from build123d import *

# Parameters (mm, degrees)
SKETCH1_R           = 32
SKETCH1_R_2         = 6
BOSS_EXTRUDE1_DEPTH = 0.3


with BuildPart() as part:
    # Sketch1 → Boss-Extrude1 (new body)
    with BuildSketch(Plane(origin=(0, 0, 0), x_dir=(1, 0, 0), z_dir=(0, 1, 0))):
        Circle(SKETCH1_R)
        Circle(SKETCH1_R_2, mode=Mode.SUBTRACT)
        with BuildLine():
            ThreePointArc((0, 25.5), (-25.112597702, 4.428028531), (-8.721513655, -23.96216183))
            ThreePointArc((-8.721513655, -23.96216183), (-8.080657273, -23.663325591), (-8.379493511, -23.022469209))
            ThreePointArc((-8.379493511, -23.022469209), (-24.127789949, 4.254380353), (0, 24.5))
            ThreePointArc((0, 24.5), (0.5, 25), (0, 25.5))
        make_face(mode=Mode.SUBTRACT)
        with BuildLine():
            ThreePointArc((18.5, 0), (3.212491287, 18.218943431), (-17.384313485, 6.327372652))
            ThreePointArc((-17.384313485, 6.327372652), (-17.085477246, 5.686516269), (-16.444620864, 5.985352508))
            ThreePointArc((-16.444620864, 5.985352508), (3.038843109, 17.234135678), (17.5, 0))
            ThreePointArc((17.5, 0), (18, -0.5), (18.5, 0))
        make_face(mode=Mode.SUBTRACT)
        with BuildLine():
            ThreePointArc((0, -25.5), (25.112597702, -4.428028531), (8.721513655, 23.96216183))
            ThreePointArc((8.721513655, 23.96216183), (8.080657273, 23.663325591), (8.379493511, 23.022469209))
            ThreePointArc((8.379493511, 23.022469209), (24.127789949, -4.254380353), (0, -24.5))
            ThreePointArc((0, -24.5), (-0.5, -25), (0, -25.5))
        make_face(mode=Mode.SUBTRACT)
        with BuildLine():
            ThreePointArc((0, 11.5), (-11.32528916, 1.996954043), (-3.933231648, -10.806465139))
            ThreePointArc((-3.933231648, -10.806465139), (-3.292375266, -10.5076289), (-3.591211505, -9.866772518))
            ThreePointArc((-3.591211505, -9.866772518), (-10.340481407, 1.823305866), (0, 10.5))
            ThreePointArc((0, 10.5), (0.5, 11), (0, 11.5))
        make_face(mode=Mode.SUBTRACT)
        with BuildLine():
            ThreePointArc((0, -11.5), (11.32528916, -1.996954043), (3.933231648, 10.806465139))
            ThreePointArc((3.933231648, 10.806465139), (3.292375266, 10.5076289), (3.591211505, 9.866772518))
            ThreePointArc((3.591211505, 9.866772518), (10.340481407, -1.823305866), (0, -10.5))
            ThreePointArc((0, -10.5), (-0.5, -11), (0, -11.5))
        make_face(mode=Mode.SUBTRACT)
        with BuildLine():
            ThreePointArc((-18.5, 0), (-3.212491287, -18.218943431), (17.384313485, -6.327372652))
            ThreePointArc((17.384313485, -6.327372652), (17.085477246, -5.686516269), (16.444620864, -5.985352508))
            ThreePointArc((16.444620864, -5.985352508), (-3.038843109, -17.234135678), (-17.5, 0))
            ThreePointArc((-17.5, 0), (-18, 0.5), (-18.5, 0))
        make_face(mode=Mode.SUBTRACT)
    extrude(amount=BOSS_EXTRUDE1_DEPTH)


solid = part.part
Input: part model. Units: mm. Frame: model coordinates. A direction names the side the tool comes from. Give positions to 0.01 mm unless a question says otherwise; leave off trailing zeros. Write each loop counter-clockwise with the first axis right and the second up, starting at its lowest first coordinate (ties: lowest second). Pieces come first, ordered by that corner, then holes.
Q1. Pull-direction query (Z, two-part tool) for faces 3 (the face through (7, 0.3, 0)), 4 (the face through (-4.76, 0.15, 3.65)), 5 (the face through (-6.94, 0.15, 31.24)); classes: pulls with the +Z half, pulls with the -Z half, needs draft (parallel to the pull), parting line crosses it, or undercut.
Q2. Section D-D, the plane x = 22. Output: boundary loops of the cut face in (y, z).
Q3. Section B-B, the plane x = 14. Output: boundary loops of the cut face in (y, z).
Q4. Section C-C, the plane y = 0.05. Output: boundary loops of the cut face in (x, z).
Q5. Material intervals for probe 1 along X at (y, z) = (0.2, -16); probe 2 along X at (y, z) = (0.2, -13); probe 3 along Z at (x, y) = (-7, 0.1), sorted ascending.
Q6. Section A-A, the plane z = -8.5. Output: boundary loops of the cut face in (x, y), plus the area to 3 significant figures.
Q7. Set-up query: faces 1 (the face through (-25.02, 0.15, -4.92)), 2 (the face through (7, 0, 0)). Return all of +Z, -Z, +X, -X, +Y, -Y with unobstructed straight access to the full face (end or side cutting, diameter ignored); none if empty.
Filled in:
1. face 3: needs draft
1. face 4: undercut
1. face 5: parting line crosses it
2. outline: (0, -23.24) - (0.3, -23.24) - (0.3, -12.89) - (0, -12.89) - close; (0, -10.78) - (0.3, -10.78) - (0.3, 10.78) - (0, 10.78) - close; (0, 12.89) - (0.3, 12.89) - (0.3, 23.24) - (0, 23.24) - close
3. outline: (0, -28.77) - (0.3, -28.77) - (0.3, -21.31) - (0, -21.31) - close; (0, -20.11) - (0.3, -20.11) - (0.3, -12.09) - (0, -12.09) - close; (0, -10.5) - (0.3, -10.5) - (0.3, 10.5) - (0, 10.5) - close; (0, 12.09) - (0.3, 12.09) - (0.3, 20.11) - (0, 20.11) - close; (0, 21.31) - (0.3, 21.31) - (0.3, 28.77) - (0, 28.77) - close
4. outline: circle Ø64 at (0, 0); hole (-18.5, 0) arc R0.5 ccw to (-17.5, 0) arc R17.5 cw to (16.44, 5.99) arc R0.5 ccw to (17.38, 6.33) arc R18.5 ccw to start; hole (-17.38, -6.33) arc R18.5 ccw to (18.5, 0) arc R0.5 ccw to (17.5, 0) arc R17.5 cw to (-16.44, -5.99) arc R0.5 ccw to start; hole (-8.72, 23.96) arc R25.5 ccw to (0, -25.5) arc R0.5 ccw to (0, -24.5) arc R24.5 cw to (-8.38, 23.02) arc R0.5 ccw to start; hole circle Ø12 at (0, 0); hole (-3.93, 10.81) arc R11.5 ccw to (0, -11.5) arc R0.5 ccw to (0, -10.5) arc R10.5 cw to (-3.59, 9.87) arc R0.5 ccw to start; hole (0, 10.5) arc R10.5 cw to (3.59, -9.87) arc R0.5 ccw to (3.93, -10.81) arc R11.5 ccw to (0, 11.5) arc R0.5 ccw to start; hole (0, 24.5) arc R24.5 cw to (8.38, -23.02) arc R0.5 ccw to (8.72, -23.96) arc R25.5 ccw to (0, 25.5) arc R0.5 ccw to start
5. probe 1: x = -27.71 to -19.86, -18.55 to -9.29, -7.09 to 7.09, 9.29 to 18.55, 19.86 to 27.71
5. probe 2: x = -29.24 to -21.94, -20.77 to -13.16, -11.72 to 11.72, 13.16 to 20.77, 21.94 to 29.24
5. probe 3: z = -31.22 to -24.52, -23.48 to -17.12, -16.04 to -9.12, -7.83 to 7.83, 9.12 to 16.04, 17.12 to 31.22
6. outline: (-30.85, 0) - (-24.04, 0) - (-24.04, 0.3) - (-30.85, 0.3) - close; (-22.98, 0) - (-16.43, 0) - (-16.43, 0.3) - (-22.98, 0.3) - close; (-15.3, 0) - (-7.75, 0) - (-7.75, 0.3) - (-15.3, 0.3) - close; (-6.16, 0) - (6.16, 0) - (6.16, 0.3) - (-6.16, 0.3) - close; (7.75, 0) - (15.3, 0) - (15.3, 0.3) - (7.75, 0.3) - close; (16.43, 0) - (22.98, 0) - (22.98, 0.3) - (16.43, 0.3) - close; (24.04, 0) - (30.85, 0) - (30.85, 0.3) - (24.04, 0.3) - close
6. area: 16.2 mm2
7. face 1: +Y, -Y
7. face 2: +Z, -Z, +X, -X, -Y
